from build123d import *

# Parameters (mm, degrees)
SM_START               = -3
SM_BASE_FLANGE_1_DEPTH = 6
SKETCH_6_R             = 9
SKETCH_6_R_2           = 68.5
CUT_EXTRUDE_1_DEPTH    = 248.757946391
FILLET_1_R             = 10


# Read off the part's stored shape, not the designer's step: Базовая кромка1
with BuildPart() as part:
    # Базовая кромка1 outline → Базовая кромка1 (new body)
    with BuildSketch(Plane(origin=(0, 0, 0), x_dir=(0, 0, -1), z_dir=(1, 0, 0)).offset(SM_START)):
        with BuildLine():
            Line((168, -14), (168, 150))
            Line((168, 150), (-168, 150))
            Line((-168, 150), (-168, -14))
            ThreePointArc((-168, -14), (0, -182), (168, -14))
        make_face()
    extrude(amount=SM_BASE_FLANGE_1_DEPTH)

    # Эскиз6 → Вырез-Вытянуть1 (cut, through all)
    with BuildSketch(Plane(origin=(3, 0, 0), x_dir=(0, 0, -1), z_dir=(1, 0, 0))):
        with Locations((-135.25, 115)):
            Circle(SKETCH_6_R)
        with Locations((-106.578454425, -83.268214538)):
            Circle(SKETCH_6_R)
        with Locations((0, -135.25)):
            Circle(SKETCH_6_R)
        with Locations((106.578454425, -83.268214538)):
            Circle(SKETCH_6_R)
        with Locations((135.25, 115)):
            Circle(SKETCH_6_R)
        Circle(SKETCH_6_R_2)
        with Locations((-135.25, 25)):
            Circle(SKETCH_6_R)
        with Locations((135.25, 25)):
            Circle(SKETCH_6_R)
    extrude(amount=-CUT_EXTRUDE_1_DEPTH, mode=Mode.SUBTRACT)

    # Скругление1
    fillet_1_edges = [part.edges().sort_by_distance(p)[0] for p in [
        (0, 150, -168),
        (0, 150, 168),
    ]]
    fillet(fillet_1_edges, radius=FILLET_1_R)


solid = part.part
Design review of the part built by this model. Coordinates are the model's own, in mm. Coordinates: 2 decimals unless noted, no trailing zeros. Write each loop counter-clockwise with the first axis right and the second up, starting at its lowest first coordinate (ties: lowest second). Pieces come first, ordered by that corner, then holes. Notation, with made-up numbers: (-34.75, 58) -> (14.25, 58) arc R23 ccw to (14.25, 67) -> close; hole circle Ø2 at (52.25, -0.5). An arc over 180 degrees is marked (long way). Write each question's results on one line, items separated by ' | '. Start each with the question number.
(1) The part is to be moulded in two halves that separate along Z. For faces 1 (the face through (-0.04, -181.96, 3.69)), 2 (the face through (0.042, -126.327, 1.172)), 3 (the face through (0.042, 21.553, -143.564)), 4 (the face through (0.04, 146.99, -165.15)), say which applies: pulls with the +Z half, pulls with the -Z half, needs draft (parallel to the pull), parting line crosses it, or undercut.
(2) Take a section at B-B on z = 0. Write out the cut boundary in (x, y), and give its area (3 significant figures).
(3) Take a section at D-D on x = -1.7. Give the number of separate pieces and of enclosed holes in the cut face, and give its area (3 significant figures).
(4) Clearance check with flat-ended pins moving along their axes: P1, Ø2, axis at x = -1.5, z = 64.5, coming from the -Y side; P2, Ø14.5, axis at y = -83.27, z = 106.58, coming from the -X side. State where each tip first meets the part, or that it passes through.
(5) Take a section at C-C on z = 44.5. Write out the cut boundary in (x, y), and give its area (3 significant figures).
(6) Take a section at A-A on y = 0. Write out the cut boundary in (x, z), and give its area (3 significant figures).
(7) For line 1 along Y through (x, z) = (-0.7, 0); line 2 along Y through (x, z) = (-2, -1.5); line 3 along Y through (x, z) = (2.65, 50.5), list the stretches that pass through material, from the lowest coordinate up. Write a range as from..to.
Results found:
1) face 1: parting line crosses it | face 2: undercut | face 3: undercut | face 4: pulls with the -Z half
2) outline: (-3, -182) -> (3, -182) -> (3, -144.25) -> (-3, -144.25) -> close; (-3, -126.25) -> (3, -126.25) -> (3, -68.5) -> (-3, -68.5) -> close; (-3, 68.5) -> (3, 68.5) -> (3, 150) -> (-3, 150) -> close | area: 1,060 mm2
3) separate pieces: 1 | enclosed holes: 8 | area: 82,900 mm2
4) P1: stops at y = -169.54 | P2: passes through
5) outline: (-3, -176) -> (3, -176) -> (3, -52.08) -> (-3, -52.08) -> close; (-3, 52.08) -> (3, 52.08) -> (3, 150) -> (-3, 150) -> close | area: 1,330 mm2
6) outline: (-3, -168) -> (3, -168) -> (3, -68.5) -> (-3, -68.5) -> close; (-3, 68.5) -> (3, 68.5) -> (3, 168) -> (-3, 168) -> close | area: 1,190 mm2
7) line 1: y = -182..-144.25, -126.25..-68.5, 68.5..150 | line 2: y = -181.99..-144.12, -126.38..-68.48, 68.48..150 | line 3: y = -174.23..-46.28, 46.28..150
